Could you check a few things on this model? Use its own coordinates, in mm. A direction names the side the tool comes from. Give positions to 0.01 mm unless a question says otherwise; leave off trailing zeros. Loops run counter-clockwise (first coordinate to the right, second up) from the corner with the lowest first, then second, coordinate; pieces in that order, holes last. Notation, with made-up numbers: M -31.75,34 L 24.25,34 A25 ccw 24.25,52 Z; hole C 33.25,-21 d11. An arc over 180 degrees is marked long. Use a Markdown table: item, result. Add a question column.
1) Suppose I cut it at B-B on y = 118.5. List the corners of the cut face in (x, z) for me, and give its area (3 significant figures).
2) If I drill on line 1 along Z through (x, y) = (1.5, 347); line 2 along Y through (x, z) = (3.5, 71.5); line 3 along Y through (x, z) = (0.5, -127), over which ranges is the centre line in solid material (lowest first)? Write a range as [from, to].
3) Suppose I cut it at C-C on z = 32.5. List the corners of the cut face in (x, y) for me, and give its area (3 significant figures).
4) Will these pins go through, and if not, where does the flat tip stop? pin 1 Ø1.9 at (x, y) = (3, 233.5) entering from +Z; pin 2 Ø1 at (x, z) = (2.5, 49.5) entering from -Y; pin 3 Ø1.9 at (x, y) = (4, 162.5) entering from +Z.
5) Suppose I cut it at A-A on x = 5.25. Count the separate pieces of the cut face and the enclosed holes in it, and give its area (3 significant figures).
6) Which directions (+Z, -Z, +X, -X, +Y, -Y) give clear straight access to the entire face, cutting with the end or side of a thin tool? Please do faces 4 (the flat face through (3.13, 159.34, -13.94)), 5 (the flat face through (0, 212, -72)), 6 (the flat face through (3.219, 329.375, 42.731)).
7) We'd pull the mould along Y, two halves only. Please class faces 1 (the flat face through (3.219, 365.623, 41.229)), 2 (the flat face through (6.35, 212, -72)), 3 (the flat face through (3.13, 360.77, -132.37)): +Y half, -Y half, draft (parallel to the pull), parting line (faces both ways), or undercut.
```python
from build123d import *

# Parameters (mm, degrees)
BOSS_EXTRUDE1_DEPTH = 6.35
SKETCH2_W           = 19.05
SKETCH2_H           = 84.666666666
SKETCH2_H_2         = 84.666666667
CUT_EXTRUDE4_DEPTH  = 7.35
FILLET1_R           = 12.7
SKETCH3_R           = 4
CUT_EXTRUDE5_DEPTH  = 7.35


with BuildPart() as part:
    # Sketch1 → Boss-Extrude1 (new body)
    with BuildSketch(Plane(origin=(0, 0, 0), x_dir=(0, 0, -1), z_dir=(1, 0, 0))):
        Polygon((-138.117194795, 324.971426047), (27.166192695, 310.511003372), (0.338937449, 3.874072765), (44.619791779, 0), (104.922607749, 0), (104.922607749, 280.894117647), (155.722607749, 304.8), (155.722607749, 311.15), (104.922607749, 419.1), (36.666498884, 419.1), (-137.563755829, 331.29726238), align=None)
    extrude(amount=BOSS_EXTRUDE1_DEPTH)

    # Sketch2 → Cut-Extrude4 (cut, through all)
    with BuildSketch(Plane(origin=(6.35, 0, 0), x_dir=(0, 0, -1), z_dir=(1, 0, 0))):
        Polygon((-102.740376399, 334.624867423), (22.028376277, 397.501651207), (15.621397962, 324.269553971), align=None)
        Polygon((87.678193652, 397.501651207), (81.234509121, 323.85), (135.710176178, 323.85), (101.05057561, 397.501651207), align=None)
        Polygon((78.456744054, 292.1), (73.172607749, 231.702045651), (73.172607749, 207.433333333), (92.222607749, 207.433333333), (92.222607749, 292.1), align=None)
        with Locations((82.697607749, 152.4)):
            Rectangle(SKETCH2_W, SKETCH2_H)
        with Locations((82.697607749, 55.033333334)):
            Rectangle(SKETCH2_W, SKETCH2_H_2)
    extrude(amount=-CUT_EXTRUDE4_DEPTH, mode=Mode.SUBTRACT)

    # Fillet1
    fillet1_edges = [part.edges().sort_by_distance(p)[0] for p in [
        (3.175, 419.1, -104.922607749),
    ]]
    fillet(fillet1_edges, radius=FILLET1_R)

    # Sketch3 → Cut-Extrude5 (cut, through all)
    with BuildSketch(Plane(origin=(6.35, 0, 0), x_dir=(0, 0, -1), z_dir=(1, 0, 0))):
        with Locations((96.863117355, 406.4)):
            Circle(SKETCH3_R)
    extrude(amount=-CUT_EXTRUDE5_DEPTH, mode=Mode.SUBTRACT)


solid = part.part
```
Answer block:
| question | item | result |
|---|---|---|
| 1 | outline | M 0,-104.92 L 6.35,-104.92 L 6.35,-92.22 L 0,-92.22 Z; M 0,-73.17 L 6.35,-73.17 L 6.35,-10.37 L 0,-10.37 Z |
| 1 | area | 479 mm^2 |
| 2 | line 1 | z = [-138.85, -124.82], [-83.26, -17.61], [78.18, 106.4] |
| 2 | line 2 | y = [319.14, 331.89], [350.37, 364.59] |
| 2 | line 3 | y = [291.28, 323.85], [342.36, 372.19] |
| 3 | outline | M 0,315.73 L 6.35,315.73 L 6.35,328.48 L 0,328.48 Z; M 0,370.02 L 6.35,370.02 L 6.35,384.24 L 0,384.24 Z |
| 3 | area | 171 mm^2 |
| 4 | pin 1 | stops at z = -20.35 |
| 4 | pin 2 | stops at y = 317.17 |
| 4 | pin 3 | stops at z = -14.13 |
| 5 | separate pieces | 1 |
| 5 | enclosed holes | 6 |
| 5 | area | 37,800 mm^2 |
| 6 | face 4 | +Z, +X, -X |
| 6 | face 5 | +Z, -Z, -X, +Y, -Y |
| 6 | face 6 | +X, -X |
| 7 | face 1 | undercut |
| 7 | face 2 | draft |
| 7 | face 3 | +Y half |
